```python
from build123d import *

# Parameters (mm, degrees)
SKETCH2_R          = 1.65
CUT_EXTRUDE1_DEPTH = 42.797129088


with BuildPart() as part:
    # Sketch1 → Revolve1 (revolve)
    with BuildSketch(Plane.XY, mode=Mode.PRIVATE) as revolve1_sk:
        Polygon((10, 0), (10, 6), (24, 6), (27, 9), (27, 14), (24, 17), (3, 17), (3, 0), align=None)
    revolve(revolve1_sk.sketch.rotate(Axis((0, 0, 0), (0, 1, 0)), 90), axis=Axis((0, 0, 0), (0, 1, 0)))

    # Sketch2 → Cut-Extrude1 (cut, through all)
    with BuildSketch(Plane.XY):
        with Locations(Location((0, 3, 0), (0, 0, 90))):
            Circle(SKETCH2_R)
    extrude(amount=-CUT_EXTRUDE1_DEPTH, mode=Mode.SUBTRACT)


solid = part.part
```
The listing builds one solid part. Answer for the finished solid, in the listing's coordinates (mm). A direction names the side the tool comes from. Round coordinates to 2 decimals unless told otherwise and drop trailing zeros. Write each loop counter-clockwise with the first axis right and the second up, starting at its lowest first coordinate (ties: lowest second). Pieces come first, ordered by that corner, then holes. Notation, with made-up numbers: (80.25, 75.5) -> (130.25, 75.5) arc R31 cw to (130.25, 99.5) -> close; hole circle Ø6 at (7, 4). An arc over 180 degrees is marked (long way). Use CSV: the item, a comma, the result in double quotes. Start each with the question number.
(1) Each of these flat-tipped pins is pushed along its axis until it touches: pin 1 (4 mm diameter, centred on y = 5.5, z = 9.5, fed in from -X); pin 2 (6 mm diameter, centred on y = 4, z = -21.5, fed in from -X); pin 3 (1.5 mm diameter, centred on x = -4.5, y = 10, fed in from -Z). Where does it stop, or does it pass through?
(2) Section B-B on z = 0 is taken. Give the vertices of the cut face in (x, y).
(3) Section D-D on y = 3 is taken. Give the vertices of the cut face in (x, z).
(4) Consider L1, parallel to X at y = 9.25, z = 0; L2, parallel to X at y = 4.5, z = 0; L3, parallel to Y at x = -7, z = -19. Determine where each line is inside the solid, lowest interval first. Write a range as from..to.
(5) Section C-C on y = 11.25 is taken. Give the vertices of the cut face in (x, z), then the cut area to 3 significant figures.
(6) Section A-A on x = 0 is taken. Give the vertices of the cut face in (y, z), then the cut area to 3 significant figures.
(7) The mould has two halves that part along X. Classify faces 3 (the face through (-0.07, 1.35, -6.2)), 4 (the face through (23.612, 6.188, 5.243)), 5 (the face through (-2.4, 0, 2.1)): released by +X, released by -X, zero draft, split by the parting line, or undercut.
(8) Which of the six approach directions +Z, -Z, +X, -X, +Y, -Y give full straight-line access (tool end or side, diameter ignored) to faces 1 (the face through (-0.3, 6, 10.3)), 2 (the face through (26.36, 11.54, 5.85))?
A:
1,pin 1,"stops at x = -23.8"
1,pin 2,"stops at x = -14.4"
1,pin 3,"stops at z = -26.74"
2,outline,"(-27, 9) -> (-24, 6) -> (-10, 6) -> (-10, 0) -> (-3, 0) -> (-3, 17) -> (-24, 17) -> (-27, 14) -> close; (3, 0) -> (10, 0) -> (10, 6) -> (24, 6) -> (27, 9) -> (27, 14) -> (24, 17) -> (3, 17) -> close"
3,outline,"(-1.65, -9.86) -> (-1.65, -2.51) arc R3 cw (long way) to (1.65, -2.51) -> (1.65, -9.86) arc R10 ccw (long way) to start"
4,L1,"x = -27..-3, 3..27"
4,L2,"x = -10..-3, 3..10"
4,L3,"y = 6..17"
5,outline,"circle Ø54 at (0, 0); hole circle Ø6 at (0, 0)"
5,area,"2,260 mm²"
6,outline,"(0, -10) -> (1.35, -10) -> (1.35, -3) -> (0, -3) -> close; (0, 3) -> (17, 3) -> (17, 24) -> (14, 27) -> (9, 27) -> (6, 24) -> (6, 10) -> (0, 10) -> close; (4.65, -10) -> (6, -10) -> (6, -24) -> (9, -27) -> (14, -27) -> (17, -24) -> (17, -3) -> (4.65, -3) -> close"
6,area,"571 mm²"
7,face 3,"undercut"
7,face 4,"split by the parting line"
7,face 5,"zero draft"
8,face 1,"-Y"
8,face 2,"+Y, -Y"
